CAD build for the part. Positions are in the model's coordinates, mm. Round coordinates to 2 decimals unless told otherwise and drop trailing zeros. Order: outer loops, then holes, each group sorted by start corner. A loop starts at its lowest first (then second) coordinate and runs counter-clockwise, first axis right, second up. Notation, with made-up numbers: M 78.5,-38 L 99.5,-38 A31 cw 99.5,-1 Z; hole C -7.5,-38 d11. An arc over 180 degrees is marked long. Put each result on its own line as item: value.
Autodesk Inventor part; units mm, degrees
ref_plane "YZ Plane" through (0, 0, 0) normal (1, 0, 0) x (0, 1, 0)
ref_plane "XZ Plane" through (0, 0, 0) normal (0, 1, 0) x (-1, 0, 0)
ref_plane "XY Plane" through (0, 0, 0) normal (0, 0, 1) x (1, 0, 0)
sketch "Sketch1" plane through (0, 0, 0) normal (0, 0, 1) x (1, 0, 0)
  line L0 (333.7348, 152.4) -> (333.7348, 508)
  line L1 (92.4348, 152.4) -> (92.4348, 419.1)
  line L2 (92.4348, 419.1) -> (301.9848, 419.1)
  line L3 (301.9848, 419.1) -> (301.9848, 152.4)
  line L4 (301.9848, 152.4) -> (333.7348, 152.4)
  line L5 (92.4348, 152.4) -> (60.6848, 152.4)
  line L6 (60.6848, 152.4) -> (60.6848, 508)
  line L7 (333.7348, 508) -> (60.6848, 508)
  point P0 (0, 0)
  point P1 (197.2098, 304.8)
  point P2 (197.2098, 442.341)
  point P3 (78.0958, 373.5705)
  point P4 (78.0958, 236.0295)
  point P5 (197.2098, 167.259)
  point P6 (316.3238, 236.0295)
  point P7 (316.3238, 373.5705)
  point P8 (311.5098, 304.8)
  point P9 (311.5098, 431.8)
  point P10 (82.9098, 431.8)
  point P11 (82.9098, 304.8)
  point P12 (235.3098, 431.8)
  point P13 (159.1098, 431.8)
  dimension "d1" = 355.6
  dimension "d4" = 137.541
  dimension "d7" = 360
  dimension "d9" = 31.75
  dimension "d21" = 31.75
  dimension "d23" = 114.3
  dimension "d39" = 127
  dimension "d40" = 127
  dimension "d48" = 22.225
  dimension "d49" = 22.225
  dimension "d54" = 209.55
  dimension "d55" = 266.7
  dimension "d56" = 104.775
  dimension "d57" = 152.4
  dimension "d58" = 152.4
extrude "Extrusion1" add sketch "Sketch1" against normal blind 3.175
hole "Hole1" at (197.2098, 304.8, 0) at (197.2098, 442.341, 0) at (78.0958, 373.5705, 0) at (78.0958, 236.0295, 0) at (197.2098, 167.259, 0) at (316.3238, 236.0295, 0) at (316.3238, 373.5705, 0) direction (0, 0, -1) diameter 6.35 depth 25.4 tip angle 118
hole "Hole3" at (311.5098, 304.8, 0) at (311.5098, 431.8, 0) at (82.9098, 431.8, 0) at (82.9098, 304.8, 0) at (159.1098, 431.8, 0) at (235.3098, 431.8, 0) direction (0, 0, -1) diameter 6.35 depth 25.4 tip angle 118
properties part number "top mid-pivot plate"
Item 1: Band-saw the part on A-A on y = 183. Give the cut face in (x, z) (3 decimals).
Answers below:
outline: M 60.685,-3.175 L 92.435,-3.175 L 92.435,0 L 60.685,0 Z; M 301.985,-3.175 L 333.735,-3.175 L 333.735,0 L 301.985,0 Z
Item 2: Band-saw the part on C-C on x = 113.5. Give the cut face in (y, z) (3 decimals), and give its area (3 significant figures).
Answers below:
outline: M 419.1,-3.175 L 508,-3.175 L 508,0 L 419.1,0 Z
area: 282 mm²
Item 3: Band-saw the part on B-B on z = -1.4. State how many separate pieces and enclosed holes the cut face has, and give its area (3 significant figures).
Answers below:
separate pieces: 1
enclosed holes: 11
area: 40,900 mm²
Item 4: Probe line 1 along X through (y, z) = (304.8, -0.9); line 2 along X through (y, z) = (323, -1.2); line 3 along X through (y, z) = (431.8, -1.7). List the from-to ranges inside material, lowest first. Write a range as [from, to].
Answers below:
line 1: [60.68, 79.73], [86.08, 92.43], [301.98, 308.33], [314.68, 333.73]
line 2: [60.68, 92.43], [301.98, 333.73]
line 3: [60.68, 79.73], [86.08, 155.93], [162.28, 232.13], [238.48, 308.33], [314.68, 333.73]
Item 5: Pin check, flat tips, straight feed: P1, Ø7.5, axis at x = 316.32, y = 236.03, coming from the +Z side; P2, Ø1, axis at x = 174.5, z = -1, coming from the -Y side. Stop position of each tip, or through.
Answers below:
P1: z = 0
P2: y = 419.1
